Can you work these out from the model? Positions are in its coordinate system, mm. Face numbers are marked on the shaded views. A direction names the side the tool comes from. Round coordinates to 2 decimals unless told otherwise and drop trailing zeros. Loops run counter-clockwise (first coordinate to the right, second up) from the corner with the lowest first, then second, coordinate; pieces in that order, holes last.
(1) I want a section at A-A on z = 1. Write out the boundary of the cut face in (x, y) (3 decimals).
(2) Which directions (+Z, -Z, +X, -X, +Y, -Y) give clear straight access to the entire face, cutting with the end or side of a thin tool? Please do the marked faces 1, 2 and 3.
(3) If I drill on line 1 along X through (y, z) = (12, -4) (3 decimals); line 2 along Y through (x, z) = (2, 1.25) (3 decimals); line 3 along Z through (x, y) = (-1, 8.5), over which ranges is the centre line in solid material (lowest first)?
(4) Thinking about a two-plate mould opening in Y: for the marked faces 4, 5 and 6, which applies, released by +Y, released by -Y, zero draft, split by the parting line, or undercut?
(5) I want a section at D-D on z = 6.25. Write out the boundary of the cut face in (x, y).
(6) I want a section at C-C on x = -0.75. Write out the boundary of the cut face in (y, z) (3 decimals).
(7) Will this pin go through, and if not, where does the flat tip stop? pin 1 Ø7 at (x, y) = (1.5, 0) entering from -Z.
(8) I want a section at B-B on y = -0.5. Write out the boundary of the cut face in (x, z) (3 decimals).
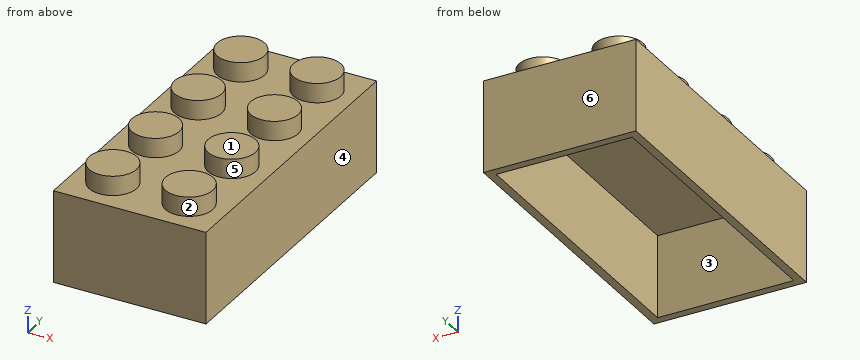
from build123d import *

# Parameters (mm, degrees)
F0_W     = 15.75
F0_H     = 9.5
F1_DEPTH = 15.875
F2_R     = 2.45
F3_DEPTH = 2
F4_W     = 14.05
F4_H     = 30.05
F5_DEPTH = 8.5


with BuildPart() as f1:
    # F0 (on Front) → F1 (new body, symmetric)
    with BuildSketch(Plane.XZ):
        Rectangle(F0_W, F0_H)
    extrude(amount=F1_DEPTH, both=True)

    # F2 (on face) → F3 (join)
    with BuildSketch(Plane.XY.offset(4.75)):
        with Locations((-3.9375, 11.90625)):
            Circle(F2_R)
        with Locations((3.9375, 11.90625)):
            Circle(F2_R)
        with Locations((3.9375, 3.96875)):
            Circle(F2_R)
        with Locations((-3.9375, 3.96875)):
            Circle(F2_R)
        with Locations((-3.9375, -3.96875)):
            Circle(F2_R)
        with Locations((3.9375, -3.96875)):
            Circle(F2_R)
        with Locations((-3.9375, -11.90625)):
            Circle(F2_R)
        with Locations((3.9375, -11.90625)):
            Circle(F2_R)
    extrude(amount=F3_DEPTH)

    # F4 (on face) → F5 (cut)
    with BuildSketch(Plane(origin=(0, 0, -4.75), x_dir=(1, 0, 0), z_dir=(0, 0, -1))):
        Rectangle(F4_W, F4_H)
    extrude(amount=-F5_DEPTH, mode=Mode.SUBTRACT)


solid = f1.part
Filled sheet:
1. outline: (-7.875, -15.875) - (7.875, -15.875) - (7.875, 15.875) - (-7.875, 15.875) - close; hole (-7.025, -15.025) - (7.025, -15.025) - (7.025, 15.025) - (-7.025, 15.025) - close
2. face 1: +Z, +X, -X, +Y, -Y
2. face 2: +Z
2. face 3: -Z
3. line 1: x = -7.875 to -7.025, 7.025 to 7.875
3. line 2: y = -15.875 to -15.025, 15.025 to 15.875
3. line 3: z = 3.75 to 4.75
4. face 4: zero draft
4. face 5: undercut
4. face 6: released by +Y
5. outline: circle Ø4.9 at (-3.94, -11.91); circle Ø4.9 at (-3.94, -3.97); circle Ø4.9 at (-3.94, 3.97); circle Ø4.9 at (-3.94, 11.91); circle Ø4.9 at (3.94, -11.91); circle Ø4.9 at (3.94, -3.97); circle Ø4.9 at (3.94, 3.97); circle Ø4.9 at (3.94, 11.91)
6. outline: (-15.875, -4.75) - (-15.025, -4.75) - (-15.025, 3.75) - (15.025, 3.75) - (15.025, -4.75) - (15.875, -4.75) - (15.875, 4.75) - (-15.875, 4.75) - close
7. pin 1: stops at z = 3.75
8. outline: (-7.875, -4.75) - (-7.025, -4.75) - (-7.025, 3.75) - (7.025, 3.75) - (7.025, -4.75) - (7.875, -4.75) - (7.875, 4.75) - (-7.875, 4.75) - close
